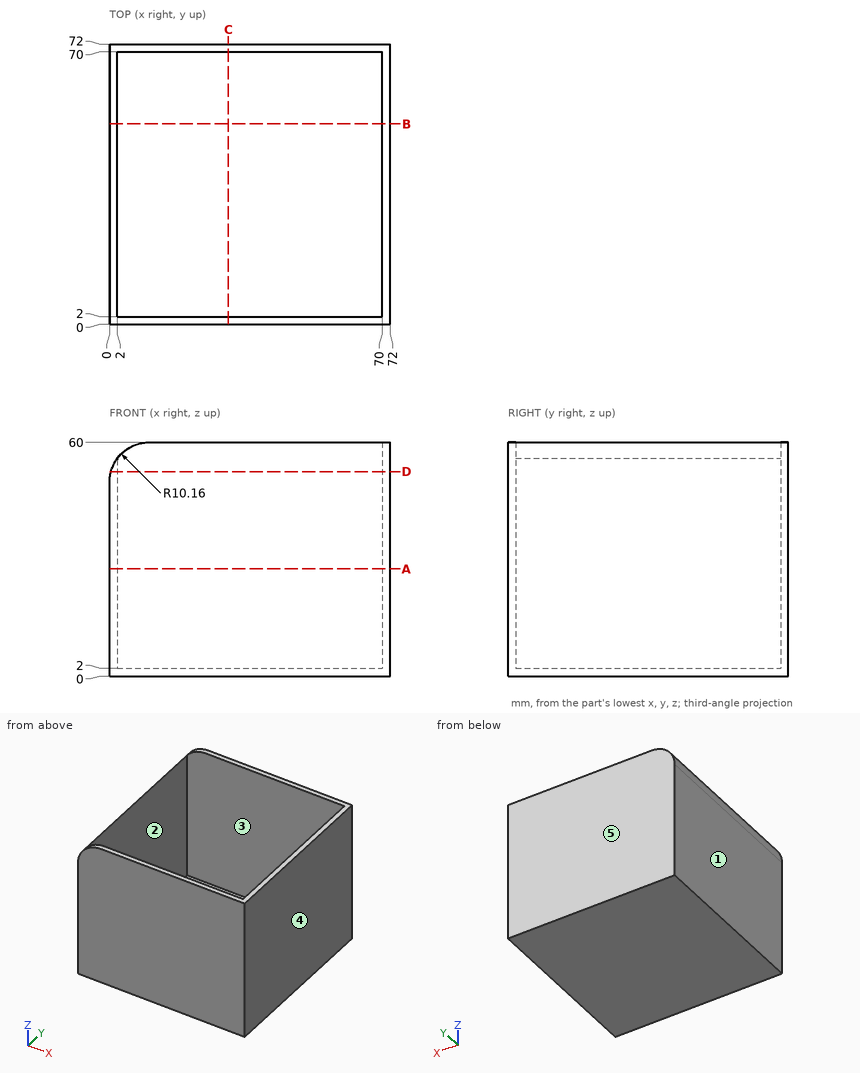
Part print with two shaded views. Sizes in mm from the minimum x, y, z corner. A direction names the side the tool comes from. Coordinates: 2 decimals unless noted, no trailing zeros. Loops run counter-clockwise (first coordinate to the right, second up) from the corner with the lowest first, then second, coordinate; pieces in that order, holes last. Notation, with made-up numbers: (11, 67.5) - (59, 67.5) arc R15 cw to (59, 82.5) - close; hole circle Ø8 at (50, 85). An arc over 180 degrees is marked (long way). Write each question's results on one line, items separated by ' | '. Start each with the question number.
Q1. Which spindle directions (+Z, -Z, +X, -X, +Y, -Y) get a long thin tool onto all of the face, cutting with end or side? Do the marked faces 1 and 2. Say none if no direction does.
Q2. Probe line 1 along X through (y, z) = (6.5, 45); line 2 along Z through (x, y) = (55.5, 53). List the from-to ranges inside material, lowest first.
Q3. Slice it at D-D on z = 52.5. Give the cut face in (x, y), and give its area (3 significant figures).
Q4. Two-plate mould, pull along X, no slides. Class the marked faces 3, 4 and 5: +X half, -X half, draft (parallel to the pull), parting line (faces both ways), or undercut.
Q5. Slice it at C-C on x = 30.5. Give the cut face in (y, z), and give its area (3 significant figures).
Q6. Slice it at A-A on z = 27.5. Give the cut face in (x, y), and give its area (3 significant figures).
Q7. Slice it at B-B on y = 51.5. Give the cut face in (x, z).
Answer:
1) face 1: +Z, -Z, -X, +Y, -Y | face 2: +Z
2) line 1: x = 0 to 2, 70 to 72 | line 2: z = 0 to 2
3) outline: (0.35, 0) - (72, 0) - (72, 72) - (0.35, 72) - close; hole (2, 2) - (70, 2) - (70, 70) - (2, 70) - close | area: 534 mm2
4) face 3: undercut | face 4: +X half | face 5: draft
5) outline: (0, 0) - (72, 0) - (72, 60) - (70, 60) - (70, 2) - (2, 2) - (2, 60) - (0, 60) - close | area: 376 mm2
6) outline: (0, 0) - (72, 0) - (72, 72) - (0, 72) - close; hole (2, 2) - (70, 2) - (70, 70) - (2, 70) - close | area: 560 mm2
7) outline: (0, 0) - (72, 0) - (72, 60) - (70, 60) - (70, 2) - (2, 2) - (2, 55.89) arc R10.16 ccw to (0, 49.84) - close
